Read the model definition and answer for the solid it produces. Units are mm, in the model's axes. A direction names the side the tool comes from. Give positions to 0.01 mm unless a question says otherwise; leave off trailing zeros. Loops run counter-clockwise (first coordinate to the right, second up) from the corner with the lowest first, then second, coordinate; pieces in that order, holes last. Notation, with made-up numbers: M -28.5,-33 L -19.5,-33 A4 ccw -19.5,-27 Z; hole C 45,74 d9. An arc over 180 degrees is marked long. Return JSON: item names as keys, results as strings. Group by question number.
```python
from build123d import *

# Parameters (mm, degrees)
F0_W     = 60
F0_H     = 70
F1_DEPTH = 2
F2_R     = 1.5
F3_W     = 2
F3_H     = 2
F4_DEPTH = 2
F5_R     = 3


with BuildPart() as f1:
    # F0 (on Top) → F1 (new body)
    with BuildSketch(Plane.XY):
        Rectangle(F0_W, F0_H)
        with BuildLine():
            ThreePointArc((-25, 27.75), (-26.5909902577, 31.5909902577), (-22.75, 30))
            Line((-22.75, 30), (22.75, 30))
            ThreePointArc((22.75, 30), (25, 32.25), (27.25, 30))
            ThreePointArc((27.25, 30), (26.5909902577, 28.4090097423), (25, 27.75))
            Line((25, 27.75), (25, -17.75))
            ThreePointArc((25, -17.75), (26.5909902577, -18.4090097423), (27.25, -20))
            ThreePointArc((27.25, -20), (25, -22.25), (22.75, -20))
            Line((22.75, -20), (-22.75, -20))
            ThreePointArc((-22.75, -20), (-26.5909902577, -21.5909902577), (-25, -17.75))
            Line((-25, -17.75), (-25, 27.75))
        make_face(mode=Mode.SUBTRACT)
        with BuildLine():
            Line((22.75, 30), (-22.75, 30))
            ThreePointArc((-22.75, 30), (-23.4090097423, 28.4090097423), (-25, 27.75))
            Line((-25, 27.75), (-25, -17.75))
            ThreePointArc((-25, -17.75), (-23.4090097423, -18.4090097423), (-22.75, -20))
            Line((-22.75, -20), (22.75, -20))
            ThreePointArc((22.75, -20), (23.4090097423, -18.4090097423), (25, -17.75))
            Line((25, -17.75), (25, 27.75))
            ThreePointArc((25, 27.75), (23.4090097423, 28.4090097423), (22.75, 30))
        make_face()
    extrude(amount=F1_DEPTH)

    # F2
    f2_edges = [f1.edges().sort_by_distance(p)[0] for p in [
        (-30, 35, 1),
        (30, 35, 1),
        (-30, -35, 1),
        (30, -35, 1),
    ]]
    fillet(f2_edges, radius=F2_R)

    # F3 (on face) → F4 (cut)
    with BuildSketch(Plane.XY.offset(2)):
        with Locations((-11.5, 6)):
            Rectangle(F3_W, F3_H)
        with Locations((-13.5, 6)):
            Rectangle(F3_W, F3_H)
        with BuildLine():
            Line((-14.5, 7), (-12.5, 7))
            Line((-12.5, 7), (-10.5, 7))
            Line((-10.5, 7), (-10.5, 12.5))
            ThreePointArc((-10.5, 12.5), (-12.5, 14.5), (-14.5, 12.5))
            Line((-14.5, 12.5), (-14.5, 7))
        make_face()
        with Locations((-11.5, 4)):
            Rectangle(F3_W, F3_H)
        with Locations((-13.5, 4)):
            Rectangle(F3_W, F3_H)
        with BuildLine():
            Line((-14.5, 5), (-14.5, 7))
            Line((-14.5, 7), (-20, 7))
            ThreePointArc((-20, 7), (-22, 5), (-20, 3))
            Line((-20, 3), (-14.5, 3))
            Line((-14.5, 3), (-14.5, 5))
        make_face()
        with BuildLine():
            Line((-5, 7), (-10.5, 7))
            Line((-10.5, 7), (-10.5, 5))
            Line((-10.5, 5), (-10.5, 3))
            Line((-10.5, 3), (-5, 3))
            ThreePointArc((-5, 3), (-3, 5), (-5, 7))
        make_face()
        with BuildLine():
            Line((-10.5, 3), (-12.5, 3))
            Line((-12.5, 3), (-14.5, 3))
            Line((-14.5, 3), (-14.5, -2.5))
            ThreePointArc((-14.5, -2.5), (-12.5, -4.5), (-10.5, -2.5))
            Line((-10.5, -2.5), (-10.5, 3))
        make_face()
        with BuildLine():
            ThreePointArc((5, 7), (3, 5), (5, 3))
            Line((5, 3), (10.5, 3))
            Line((10.5, 3), (10.5, 5))
            Line((10.5, 5), (10.5, 7))
            Line((10.5, 7), (5, 7))
        make_face()
        with Locations((11.5, 4)):
            Rectangle(F3_W, F3_H)
        with BuildLine():
            Line((12.5, 3), (10.5, 3))
            Line((10.5, 3), (10.5, -2.5))
            ThreePointArc((10.5, -2.5), (12.5, -4.5), (14.5, -2.5))
            Line((14.5, -2.5), (14.5, 3))
            Line((14.5, 3), (12.5, 3))
        make_face()
        with Locations((13.5, 4)):
            Rectangle(F3_W, F3_H)
        with Locations((11.5, 6)):
            Rectangle(F3_W, F3_H)
        with BuildLine():
            Line((10.5, 12.5), (10.5, 7))
            Line((10.5, 7), (12.5, 7))
            Line((12.5, 7), (14.5, 7))
            Line((14.5, 7), (14.5, 12.5))
            ThreePointArc((14.5, 12.5), (12.5, 14.5), (10.5, 12.5))
        make_face()
        with BuildLine():
            Line((14.5, 5), (14.5, 3))
            Line((14.5, 3), (20, 3))
            ThreePointArc((20, 3), (22, 5), (20, 7))
            Line((20, 7), (14.5, 7))
            Line((14.5, 7), (14.5, 5))
        make_face()
        with Locations((13.5, 6)):
            Rectangle(F3_W, F3_H)
    extrude(amount=-F4_DEPTH, mode=Mode.SUBTRACT)

    # F5
    f5_edges = [f1.edges().sort_by_distance(p)[0] for p in [
        (-14.5, 3, 1),
        (-10.5, 3, 1),
        (-14.5, 7, 1),
        (-10.5, 7, 1),
        (10.5, 3, 1),
        (10.5, 7, 1),
        (14.5, 3, 1),
        (14.5, 7, 1),
    ]]
    fillet(f5_edges, radius=F5_R)


solid = f1.part
```
1. Find section B-B (x = -12.5). Write down the section's boundary in (y, z), and give its area (3 significant figures).
2. Find section C-C (z = 0.4). State how many separate pieces and enclosed holes the cut face has, and give its area (3 significant figures).
3. Find section D-D (x = -4). Write down the section's boundary in (y, z).
4. For faces 4 (the flat face through (-6, 3, 1)), 5 (the flat face through (0, 0, 2)), determine the directions among +Z, -Z, +X, -X, +Y, -Y from which every point of the face is accessible in a straight line to the end or side of a thin tool.
5. Find section A-A (y = 5). Write down the section's boundary in (x, z), and give its area (3 significant figures).
6. Straight lines are drawn through the part: line 1 along X through (y, z) = (5, 0.5); line 2 along X through (y, z) = (30, 0.95); line 3 along Y through (x, z) = (-25, 0.65). For each, find the intervals that lie inside material, in ascending order.
7. The mould has two halves that part along Y. Classify faces 1 (the cylindrical face through (-29.57, -34.55, 1.01)), 2 (the cylindrical face through (9.64, 7.9, 0.99)), 3 (the flat face through (-30, 0, 1)): +Y half, -Y half, draft (parallel to the pull), parting line (faces both ways), or undercut.
Result:
{
 "1": {"outline": "M -35,0 L -4.5,0 L -4.5,2 L -35,2 Z; M 14.5,0 L 35,0 L 35,2 L 14.5,2 Z", "area": "102 mm2"},
 "2": {"separate pieces": "1", "enclosed holes": "6", "area": "3,860 mm2"},
 "3": {"outline": "M -35,0 L 3.27,0 L 3.27,2 L -35,2 Z; M 6.73,0 L 35,0 L 35,2 L 6.73,2 Z"},
 "4": {"face 4": "+Z, -Z", "face 5": "+Z, +X, -X, +Y, -Y"},
 "5": {"outline": "M -30,0 L -22,0 L -22,2 L -30,2 Z; M -3,0 L 3,0 L 3,2 L -3,2 Z; M 22,0 L 30,0 L 30,2 L 22,2 Z", "area": "44.0 mm2"},
 "6": {"line 1": "x = -30 to -22, -3 to 3, 22 to 30", "line 2": "x = -30 to -27.25, -22.75 to 22.75, 27.25 to 30", "line 3": "y = -35 to -22.25, -17.75 to 27.75, 32.25 to 35"},
 "7": {"face 1": "-Y half", "face 2": "undercut", "face 3": "draft"}
}
